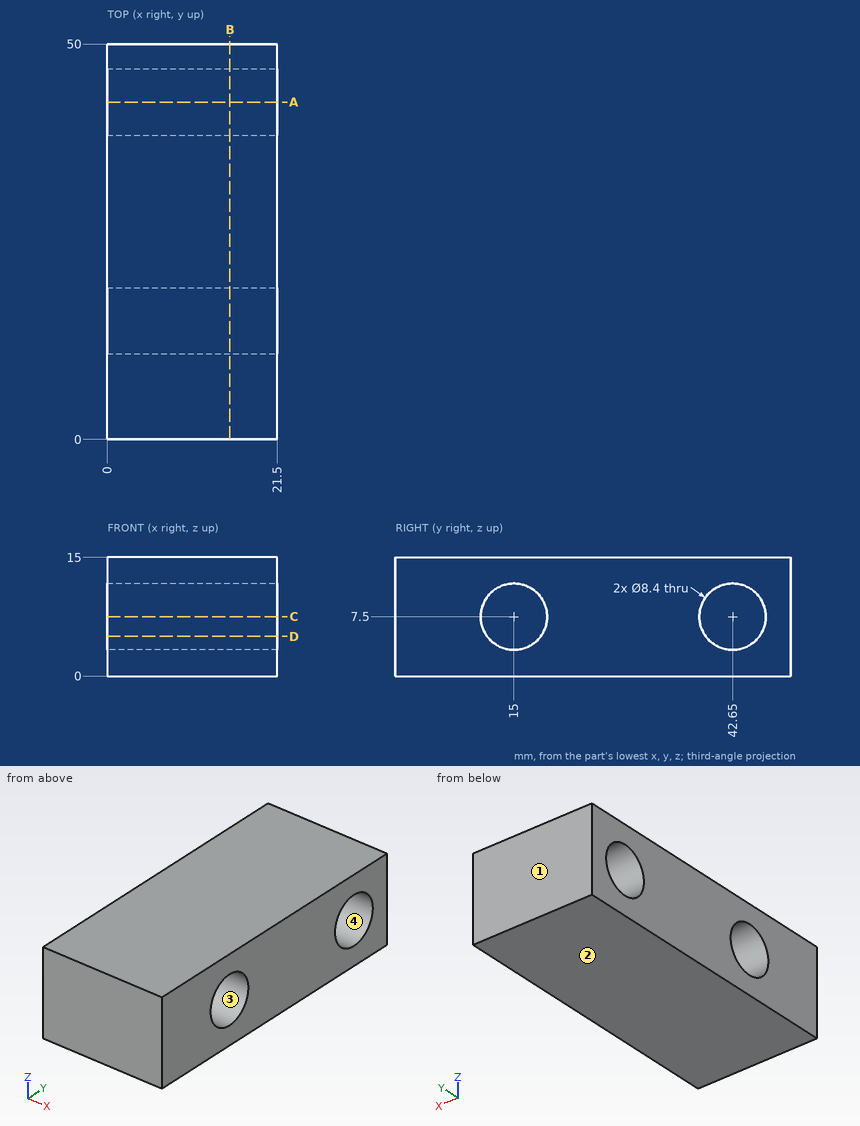
Part print with two shaded views. Sizes in mm from the minimum x, y, z corner. Coordinates: 2 decimals unless noted, no trailing zeros. Loops run counter-clockwise (first coordinate to the right, second up) from the corner with the lowest first, then second, coordinate; pieces in that order, holes last. Notation, with made-up numbers: (60.25, 15.25) -> (105.25, 15.25) arc R19 cw to (105.25, 35.25) -> close; hole circle Ø9 at (11.25, -4.5). An arc over 180 degrees is marked (long way). Answer as a JSON object with one key per item and string values.
Q1. Cut at D-D (z = 5). List the corners of the cut face in (x, y).
Report:
{"outline": "(0, 0) -> (21.5, 0) -> (21.5, 11.63) -> (0, 11.63) -> close; (0, 18.37) -> (21.5, 18.37) -> (21.5, 39.28) -> (0, 39.28) -> close; (0, 46.02) -> (21.5, 46.02) -> (21.5, 50) -> (0, 50) -> close"}
Q2. Cut at A-A (y = 42.65). List the corners of the cut face in (x, z), and give its area (3 significant figures).
Report:
{"outline": "(0, 0) -> (21.5, 0) -> (21.5, 3.3) -> (0, 3.3) -> close; (0, 11.7) -> (21.5, 11.7) -> (21.5, 15) -> (0, 15) -> close", "area": "142 mm2"}
Q3. Cut at B-B (x = 15.5). List the corners of the cut face in (y, z), and give its area (3 significant figures).
Report:
{"outline": "(0, 0) -> (50, 0) -> (50, 15) -> (0, 15) -> close; hole circle Ø8.4 at (15, 7.5); hole circle Ø8.4 at (42.65, 7.5)", "area": "639 mm2"}
Q4. Pull direction Y, two halves, no side cores. Call the marked faces 1, 2, 3 and 4: released by +Y, released by -Y, zero draft, split by the parting line, or undercut.
Report:
{"face 1": "released by +Y", "face 2": "zero draft", "face 3": "undercut", "face 4": "undercut"}
Q5. Probe probe 1 along Y at (x, z) = (9, 7.5); probe 2 along Z at (x, y) = (7, 42.65); probe 3 along Y at (x, z) = (20, 5). List the from-to ranges inside material, lowest first.
Report:
{"probe 1": "y = 0 to 10.8, 19.2 to 38.45, 46.85 to 50", "probe 2": "z = 0 to 3.3, 11.7 to 15", "probe 3": "y = 0 to 11.63, 18.37 to 39.28, 46.02 to 50"}
Q6. Cut at C-C (z = 7.5). List the corners of the cut face in (x, y), and give its area (3 significant figures).
Report:
{"outline": "(0, 0) -> (21.5, 0) -> (21.5, 10.8) -> (0, 10.8) -> close; (0, 19.2) -> (21.5, 19.2) -> (21.5, 38.45) -> (0, 38.45) -> close; (0, 46.85) -> (21.5, 46.85) -> (21.5, 50) -> (0, 50) -> close", "area": "714 mm2"}
